Verification items for the finished model (mm, model axes). Give positions to 0.01 mm unless a question says otherwise; leave off trailing zeros. Order: outer loops, then holes, each group sorted by start corner. A loop starts at its lowest first (then second) coordinate and runs counter-clockwise, first axis right, second up. Notation, with made-up numbers: (-35.5, -17.75) - (4.5, -17.75) arc R29 cw to (4.5, 3.25) - close; hole circle Ø5 at (61.5, 11.5). An arc over 180 degrees is marked (long way). Answer as a JSON object with one key per item and string values.
```python
from build123d import *

# Parameters (mm, degrees)
SKETCH1_R           = 12.7
SKETCH1_R_2         = 6.35
BOSS_EXTRUDE1_DEPTH = 3.175


with BuildPart() as part:
    # Sketch1 → Boss-Extrude1 (new body)
    with BuildSketch(Plane.XY):
        with Locations((-17.213222871, 25.742348898)):
            Circle(SKETCH1_R)
        with Locations((-17.213222871, 25.742348898)):
            Circle(SKETCH1_R_2, mode=Mode.SUBTRACT)
        with BuildLine():
            Line((-29.913222871, 25.742348898), (-29.913222871, -25.057651102))
            ThreePointArc((-29.913222871, -25.057651102), (-17.213222871, -12.357651102), (-4.513222871, -25.057651102))
            Line((-4.513222871, -25.057651102), (-4.513222871, 25.742348898))
            ThreePointArc((-4.513222871, 25.742348898), (-17.213222871, 13.042348898), (-29.913222871, 25.742348898))
        make_face()
        with Locations((-17.213222871, -25.057651102)):
            Circle(SKETCH1_R)
        with Locations((-17.213222871, -25.057651102)):
            Circle(SKETCH1_R_2, mode=Mode.SUBTRACT)
    extrude(amount=BOSS_EXTRUDE1_DEPTH)


solid = part.part
```
(1) Section check D-D (y = 29). Record the cut outline in (x, z) (3 decimals), then the cut area to 3 significant figures.
Computed values:
{"outline": "(-29.488, 0) - (-22.664, 0) - (-22.664, 3.175) - (-29.488, 3.175) - close; (-11.763, 0) - (-4.938, 0) - (-4.938, 3.175) - (-11.763, 3.175) - close", "area": "43.3 mm²"}
(2) Section check B-B (x = -16). Record the cut outline in (y, z) (3 decimals), then the cut area to 3 significant figures.
Computed values:
{"outline": "(-37.7, 0) - (-31.291, 0) - (-31.291, 3.175) - (-37.7, 3.175) - close; (-18.825, 0) - (19.509, 0) - (19.509, 3.175) - (-18.825, 3.175) - close; (31.975, 0) - (38.384, 0) - (38.384, 3.175) - (31.975, 3.175) - close", "area": "162 mm²"}
(3) Release check for a two-part mould opening along Y. For faces 1 (the cylindrical face through (-16.93, 38.44, 1.57)), 2 (the flat face through (-17, 1, 0)), 3 (the cylindrical face through (-18.59, 19.543, 1.565)) record: pulls with the +Y half, pulls with the -Y half, needs draft (parallel to the pull), parting line crosses it, or undercut.
Computed values:
{"face 1": "pulls with the +Y half", "face 2": "needs draft", "face 3": "undercut"}
(4) Material ranges on line 1 along Y through (x, z) = (-14.25, 2.3); line 2 along Y through (x, z) = (-22.25, 1.8); line 3 along X through (y, z) = (21, 0.7), recorded low to high. Write a range as [from, to].
Computed values:
{"line 1": "y = [-37.41, -30.67], [-19.44, 20.13], [31.36, 38.09]", "line 2": "y = [-36.72, -28.92], [-21.19, 21.88], [29.61, 37.4]", "line 3": "x = [-29.91, -21.44], [-12.99, -4.51]"}
(5) Section check C-C (z = 2.25). Record the cut outline in (x, y).
Computed values:
{"outline": "(-29.91, -25.06) arc R12.7 ccw to (-4.51, -25.06) - (-4.51, 25.74) arc R12.7 ccw to (-29.91, 25.74) - close; hole circle Ø12.7 at (-17.21, -25.06); hole circle Ø12.7 at (-17.21, 25.74)"}
(6) Section check A-A (y = -28). Record the cut outline in (x, z) (3 decimals).
Computed values:
{"outline": "(-29.568, 0) - (-22.84, 0) - (-22.84, 3.175) - (-29.568, 3.175) - close; (-11.586, 0) - (-4.859, 0) - (-4.859, 3.175) - (-11.586, 3.175) - close"}
